The listing builds one solid part. Answer for the finished solid, in the listing's coordinates (mm). Give positions to 0.01 mm unless a question says otherwise; leave off trailing zeros. Order: outer loops, then holes, each group sorted by start corner. A loop starts at its lowest first (then second) coordinate and runs counter-clockwise, first axis right, second up. Notation, with made-up numbers: (-23.5, 16.5) - (10.5, 16.5) arc R18 cw to (10.5, 31.5) - close; hole circle Ø3 at (9, -16). An arc over 180 degrees is marked (long way). Use CSV: the item, a comma, the result in double quotes.
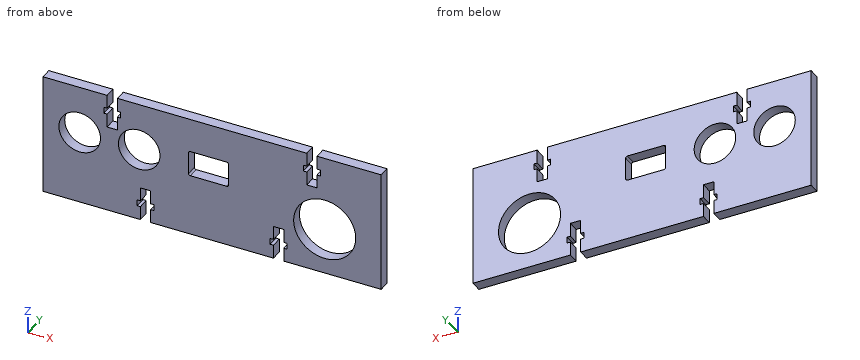
```python
from build123d import *

# Parameters (mm, degrees)
SKETCH1_W                = 96.8375
SKETCH1_H                = 34.925
BOSS_EXTRUDE1_DEPTH      = 3.175
F_7_16_CLEARANCE_HOLE1_D = 11.90498
SKETCH6_W                = 11.43
SKETCH6_H                = 7.366
CUT_EXTRUDE1_DEPTH       = 52.56932114
CUT_EXTRUDE3_DEPTH       = 52.56932114
SKETCH9_R                = 8.89
CUT_EXTRUDE4_DEPTH       = 52.56932114
FILLET1_R                = 0.508


with BuildPart() as part:
    # Sketch1 → Boss-Extrude1 (new body)
    with BuildSketch(Plane(origin=(0, 0, 0), x_dir=(1, 0, 0), z_dir=(0, 1, 0))):
        Rectangle(SKETCH1_W, SKETCH1_H)
    extrude(amount=BOSS_EXTRUDE1_DEPTH)

    # 7/16 Clearance Hole1 (through all)
    with Locations(Plane(origin=(0, 3.175, 0), x_dir=(1, 0, 0), z_dir=(0, 1, 0))):
        with Locations((-37.9095, -3.7465), (-20.8661, -3.7465)):
            Hole(F_7_16_CLEARANCE_HOLE1_D / 2)

    # Sketch6 → Cut-Extrude1 (cut, through all)
    with BuildSketch(Plane(origin=(0, 3.175, 0), x_dir=(1, 0, 0), z_dir=(0, 1, 0))):
        with Locations((-1.016, -4.0005)):
            Rectangle(SKETCH6_W, SKETCH6_H)
    extrude(amount=-CUT_EXTRUDE1_DEPTH, mode=Mode.SUBTRACT)

    # Sketch8 → Cut-Extrude3 (cut, through all)
    with BuildSketch(Plane(origin=(0, 3.175, 0), x_dir=(1, 0, 0), z_dir=(0, 1, 0))):
        Polygon((27.1018, -17.4625), (30.0482, -17.4625), (30.0482, -13.5255), (30.988, -13.5255), (30.988, -11.7475), (30.0482, -11.7475), (30.0482, -7.8105), (27.1018, -7.8105), (27.1018, -11.7475), (26.162, -11.7475), (26.162, -13.5255), (27.1018, -13.5255), align=None)
        Polygon((-30.0482, -17.4625), (-27.1018, -17.4625), (-27.1018, -13.5255), (-26.162, -13.5255), (-26.162, -11.7475), (-27.1018, -11.7475), (-27.1018, -7.8105), (-30.0482, -7.8105), (-30.0482, -11.7475), (-30.988, -11.7475), (-30.988, -13.5255), (-30.0482, -13.5255), align=None)
        Polygon((17.5768, 11.7475), (17.5768, 7.8105), (20.5232, 7.8105), (20.5232, 11.7475), (21.463, 11.7475), (21.463, 13.5255), (20.5232, 13.5255), (20.5232, 17.4625), (17.5768, 17.4625), (17.5768, 13.5255), (16.637, 13.5255), (16.637, 11.7475), align=None)
        Polygon((-20.5232, 11.7475), (-20.5232, 7.8105), (-17.5768, 7.8105), (-17.5768, 11.7475), (-16.637, 11.7475), (-16.637, 13.5255), (-17.5768, 13.5255), (-17.5768, 17.4625), (-20.5232, 17.4625), (-20.5232, 13.5255), (-21.463, 13.5255), (-21.463, 11.7475), align=None)
    extrude(amount=-CUT_EXTRUDE3_DEPTH, mode=Mode.SUBTRACT)

    # Sketch9 → Cut-Extrude4 (cut, through all)
    with BuildSketch(Plane(origin=(0, 3.175, 0), x_dir=(1, 0, 0), z_dir=(0, 1, 0))):
        with Locations(Location((32.2326, 4.1275, 0), (0, 0, 270))):
            Circle(SKETCH9_R)
    extrude(amount=-CUT_EXTRUDE4_DEPTH, mode=Mode.SUBTRACT)

    # Fillet1
    fillet1_edges = [part.edges().sort_by_distance(p)[0] for p in [
        (4.699, 1.5875, 0.3175),
        (4.699, 1.5875, 7.6835),
        (-6.731, 1.5875, 7.6835),
        (-6.731, 1.5875, 0.3175),
    ]]
    fillet(fillet1_edges, radius=FILLET1_R)


solid = part.part
```
Item 1: This flat-tipped pin is pushed along its axis until it touches: pin 1 (0.9 mm diameter, centred on x = 19, y = 1, fed in from -Z). Where does it stop, or does it pass through?
Taken from the geometry:
pin 1,"z = -7.81"
Item 2: The part is cut by section A-A (x = 39). Give the vertices of the cut face in (y, z) (1 decimal).
Taken from the geometry:
outline,"(0, -17.5) - (3.2, -17.5) - (3.2, -9.9) - (0, -9.9) - close; (0, 1.6) - (3.2, 1.6) - (3.2, 17.5) - (0, 17.5) - close"
Item 3: The part is cut by section B-B (y = 2.1). Count the separate pieces of the cut face and the enclosed holes in it, and give its area (3 significant figures).
Taken from the geometry:
separate pieces,"1"
enclosed holes,"4"
area,"2,700 mm^2"
Item 4: Find the intervals of material crossed by line 1 along X through (y, z) = (2.2, 11); line 2 along X through (y, z) = (1.1, -15); line 3 along Z through (x, y) = (2.5, 0.3), in increasing order.
Taken from the geometry:
line 1,"-48.42 to -30.05, -27.1 to 27.1, 30.05 to 48.42"
line 2,"-48.42 to -20.52, -17.58 to 17.58, 20.52 to 48.42"
line 3,"-17.46 to 0.32, 7.68 to 17.46"
